Check sheet for the modelled part. Datum: model origin and axes. Units: mm. Round coordinates to 2 decimals unless told otherwise and drop trailing zeros. Loops run counter-clockwise (first coordinate to the right, second up) from the corner with the lowest first, then second, coordinate; pieces in that order, holes last. Notation, with made-up numbers: (-35, 47) - (-12, 47) arc R26 cw to (-12, 69) - close; hole circle Ø6 at (88, -3.75). An arc over 180 degrees is marked (long way). Answer in a Markdown table with one row per item. Add a question column.
(1) Thickness scan on line 1 along Z through (x, y) = (4, -347); line 2 along Y through (x, z) = (1.5, -99); line 3 along Z through (x, y) = (4.5, 3). Record the ranges inside material, lowest first.
(2) Cross-section at A-A on y = -177.5. Enter the section's corners in (x, z), then the cut area to 3 significant figures.
(3) Cross-section at C-C on z = -163. Enter the section's corners in (x, y), then the cut area to 3 significant figures.
(4) Cross-section at B-B on x = 3. Count the separate pieces of the cut face and the enclosed holes in it, then the cut area to 3 significant figures.
(5) Gauge pin test, flat ends, axial feed: pin 1 (7.5 mm diameter, centred on y = -65.41, z = -404.06, fed in from +X); pin 2 (2 mm diameter, centred on x = 3, z = -36, fed in from +Y); pin 3 (1 mm diameter, centred on x = 4, y = -63.5, fed in from +Z); pin 4 (1 mm diameter, centred on x = 1, y = -54, fed in from +Z). Record the tip position at first contact, or that the pin passes through.
from build123d import *

# Parameters (mm, degrees)
SKETCH1_W                            = 508
SKETCH1_H                            = 609.6
BOSS_EXTRUDE1_DEPTH                  = 6.35
CUT_EXTRUDE1_DEPTH                   = 6.35
F_3_4_0_75_DIAMETER_HOLE1_AT_2_COUNT = 2
F_3_4_0_75_DIAMETER_HOLE1_AT_2_PITCH = 528.299128293
F_1_4_0_25_DIAMETER_HOLE1_D          = 6.35
LPATTERN2_OUTLINE_R                  = 3.175
LPATTERN2_DEPTH                      = 6.35


# Read off the part's stored shape, not the designer's step: LPattern2
with BuildPart() as part:
    # Sketch1 → Boss-Extrude1 (new body)
    with BuildSketch(Plane(origin=(0, 0, 0), x_dir=(0, 0, -1), z_dir=(1, 0, 0))):
        with Locations((167.525841453, -255.907437784)):
            Rectangle(SKETCH1_W, SKETCH1_H)
    extrude(amount=BOSS_EXTRUDE1_DEPTH)

    # Sketch4 → Cut-Extrude1 (cut)
    with BuildSketch(Plane(origin=(6.35, 0, 0), x_dir=(0, 0, -1), z_dir=(1, 0, 0))):
        Polygon((-86.474158547, 48.892562216), (243.725841453, 48.892562216), (-86.474158547, -332.107437784), align=None)
    extrude(amount=-CUT_EXTRUDE1_DEPTH, mode=Mode.SUBTRACT)

    # Sketch6 → 3/4 (0.75) Diameter Hole1 (revolve, cut)
    with BuildSketch(Plane(origin=(6.35, -341.632437784, 14.084158547), x_dir=(0, 0, -1), z_dir=(0, 1, 0))):
        Polygon((0, 0), (0, 6.35), (9.525, 6.35), (9.525, 0.635), (10.16, 0), align=None)
    f_3_4_0_75_diameter_hole1 = revolve(axis=Axis((12.7, -341.632437784, 14.084158547), (-1, 0, 0)), mode=Mode.SUBTRACT)

    # 3/4 (0.75) Diameter Hole1 at 2: 3/4 (0.75) Diameter Hole1 ×2
    with Locations(*[Vector(0, 0.6765499642400948, -0.7363967313118156) * (i * F_3_4_0_75_DIAMETER_HOLE1_AT_2_PITCH) for i in range(1, F_3_4_0_75_DIAMETER_HOLE1_AT_2_COUNT)]):
        add(f_3_4_0_75_diameter_hole1, mode=Mode.SUBTRACT)

    # 1/4 (0.25) Diameter Hole1 (through all)
    with Locations(Plane(origin=(6.35, 0, 0), x_dir=(0, 0, -1), z_dir=(1, 0, 0))):
        with Locations((-78.536658547, -522.607437784), (-78.536658547, -471.807437784), (-53.136658547, -522.607437784), (-53.136658547, -471.807437784), (-27.736658547, -522.607437784), (-27.736658547, -471.807437784), (-2.336658547, -522.607437784), (-2.336658547, -471.807437784), (23.063341453, -522.607437784), (23.063341453, -471.807437784), (48.463341453, -522.607437784), (48.463341453, -471.807437784), (73.863341453, -522.607437784), (73.863341453, -471.807437784), (99.263341453, -522.607437784), (99.263341453, -471.807437784), (124.663341453, -522.607437784), (124.663341453, -471.807437784), (150.063341453, -522.607437784), (150.063341453, -471.807437784), (175.463341453, -522.607437784), (175.463341453, -471.807437784), (200.863341453, -522.607437784), (200.863341453, -471.807437784), (226.263341453, -522.607437784), (226.263341453, -471.807437784), (251.663341453, -522.607437784), (251.663341453, -471.807437784), (277.063341453, -522.607437784), (277.063341453, -471.807437784), (302.463341453, -522.607437784), (302.463341453, -471.807437784), (327.863341453, -522.607437784), (327.863341453, -471.807437784), (353.263341453, -522.607437784), (353.263341453, -471.807437784), (378.663341453, -522.607437784), (378.663341453, -471.807437784), (404.063341453, -522.607437784), (404.063341453, -471.807437784)):
            Hole(F_1_4_0_25_DIAMETER_HOLE1_D / 2)

    # LPattern2 outline → LPattern2 (cut)
    with BuildSketch(Plane.YZ):
        with Locations((36.192562216, -404.063341453)):
            Circle(LPATTERN2_OUTLINE_R)
        with Locations((10.792562216, -404.063341453)):
            Circle(LPATTERN2_OUTLINE_R)
        with Locations((-14.607437784, -404.063341453)):
            Circle(LPATTERN2_OUTLINE_R)
        with Locations((-40.007437784, -404.063341453)):
            Circle(LPATTERN2_OUTLINE_R)
        with Locations((-65.407437784, -404.063341453)):
            Circle(LPATTERN2_OUTLINE_R)
        with Locations((-90.807437784, -404.063341453)):
            Circle(LPATTERN2_OUTLINE_R)
        with Locations((-116.207437784, -404.063341453)):
            Circle(LPATTERN2_OUTLINE_R)
        with Locations((-141.607437784, -404.063341453)):
            Circle(LPATTERN2_OUTLINE_R)
        with Locations((-167.007437784, -404.063341453)):
            Circle(LPATTERN2_OUTLINE_R)
        with Locations((-192.407437784, -404.063341453)):
            Circle(LPATTERN2_OUTLINE_R)
        with Locations((-217.807437784, -404.063341453)):
            Circle(LPATTERN2_OUTLINE_R)
        with Locations((-243.207437784, -404.063341453)):
            Circle(LPATTERN2_OUTLINE_R)
        with Locations((-268.607437784, -404.063341453)):
            Circle(LPATTERN2_OUTLINE_R)
        with Locations((-294.007437784, -404.063341453)):
            Circle(LPATTERN2_OUTLINE_R)
        with Locations((-319.407437784, -404.063341453)):
            Circle(LPATTERN2_OUTLINE_R)
        with Locations((-344.807437784, -404.063341453)):
            Circle(LPATTERN2_OUTLINE_R)
        with Locations((-370.207437784, -404.063341453)):
            Circle(LPATTERN2_OUTLINE_R)
        with Locations((-395.607437784, -404.063341453)):
            Circle(LPATTERN2_OUTLINE_R)
        with Locations((-421.007437784, -404.063341453)):
            Circle(LPATTERN2_OUTLINE_R)
        with Locations((-446.407437784, -404.063341453)):
            Circle(LPATTERN2_OUTLINE_R)
    extrude(amount=LPATTERN2_DEPTH, mode=Mode.SUBTRACT)


solid = part.part
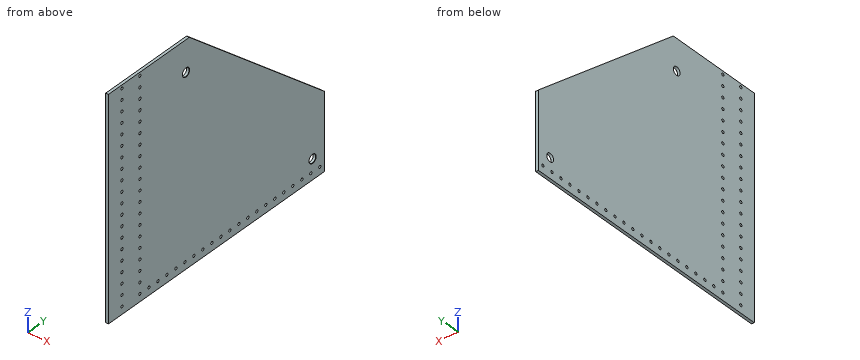
Answers:
| question | item | result |
|---|---|---|
| 1 | line 1 | z = -421.53 to -406.36, -401.77 to 6.22, 21.95 to 86.47 |
| 1 | line 2 | y = -560.71 to -525.77, -519.44 to -474.97, -468.64 to -118.1 |
| 1 | line 3 | z = -421.53 to -203.95 |
| 2 | outline | (0, -421.53) - (6.35, -421.53) - (6.35, -47.52) - (0, -47.52) - close |
| 2 | area | 2,370 mm^2 |
| 3 | outline | (0, -560.71) - (6.35, -560.71) - (6.35, -44.25) - (0, -44.25) - close |
| 3 | area | 3,280 mm^2 |
| 4 | separate pieces | 1 |
| 4 | enclosed holes | 62 |
| 4 | area | 244,000 mm^2 |
| 5 | pin 1 | stops at x = 6.35 |
| 5 | pin 2 | stops at y = -189.64 |
| 5 | pin 3 | stops at z = -145.89 |
| 5 | pin 4 | stops at z = -154.12 |
